For this review, use the dimensioned drawing (mm, ordinates from the lowest corner) and the shaded views. A direction names the side the tool comes from. Coordinates: 2 decimals unless noted, no trailing zeros. Loops run counter-clockwise (first coordinate to the right, second up) from the corner with the lowest first, then second, coordinate; pieces in that order, holes last. Notation, with made-up numbers: M 40.25,20.5 L 88.25,20.5 A30 cw 88.25,56.5 Z; hole C -39.5,41.5 d11. An arc over 180 degrees is marked long. Write item = value, one per line. Start each with the question number.
Q1. We need section D-D on z = 12.75. Give the boundary of the cut face in (x, y), and give its area (3 significant figures).
Q2. Mouldability with a two-part tool opening along Z and no side actions: class the marked faces 3 and 4 as released by +Z, released by -Z, zero draft, split by the parting line, or undercut.
Q3. We need section C-C on y = 4. Give the boundary of the cut face in (x, z), and give its area (3 significant figures).
Q4. We need section A-A on z = 8. Give the boundary of the cut face in (x, y).
Q5. We need section B-B on x = 30. Give the boundary of the cut face in (y, z).
Q6. Clearance check with flat-ended pins moving along their axes: pin 1 Ø2 at (x, z) = (11.5, 13) entering from -Y; pin 2 Ø6 at (y, z) = (27, 11.5) entering from +X; pin 3 Ø6 at (x, y) = (45, 13.5) entering from -Z. State where each tip first meets the part, or that it passes through.
Q7. Wall thickness on probe 1 along X at (y, z) = (15.5, 8); probe 2 along Y at (x, z) = (51.5, 8): over which ranges is each line inside the solid? List them lowest first.
Q8. For the marked faces 1 and 2, list the 3-axis set-ups (+Z, -Z, +X, -X, +Y, -Y) from which the entire face can be reached by the end or side of a thin tool; tool diameter is ignored.
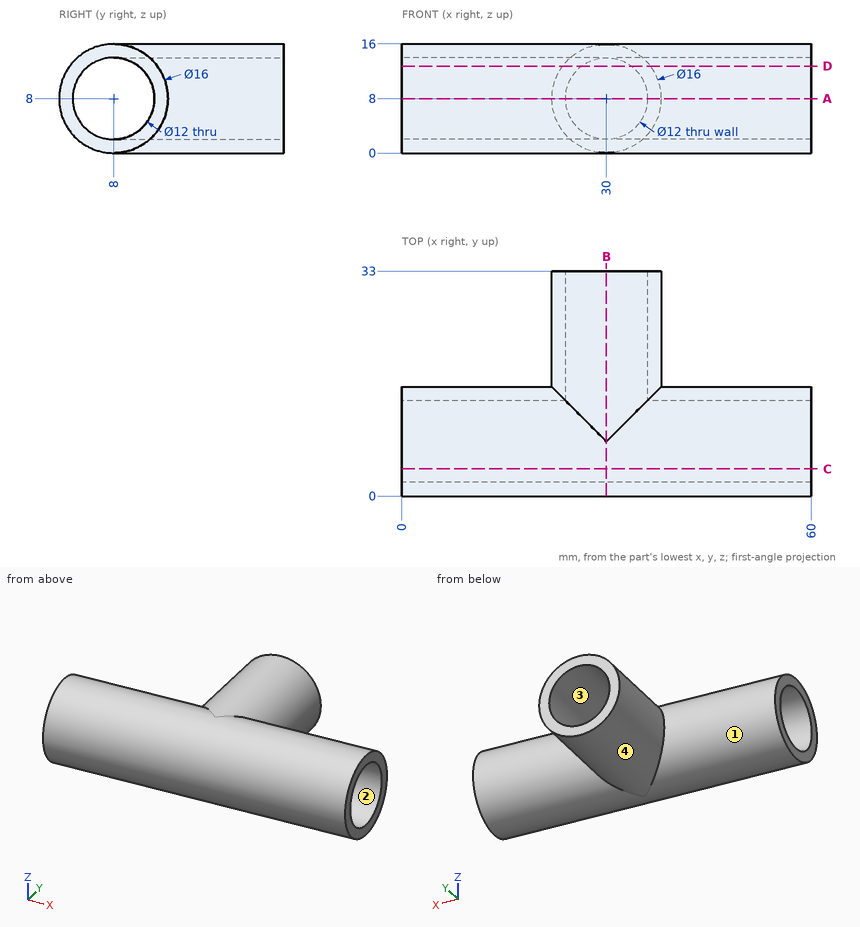
Returned:
q1.outline = M 0,1.56 L 60,1.56 L 60,4.33 L 0,4.33 Z; M 0,11.67 L 26.33,11.67 L 26.33,33 L 23.56,33 L 23.56,14.44 L 0,14.44 Z; M 33.67,11.67 L 60,11.67 L 60,14.44 L 36.44,14.44 L 36.44,33 L 33.67,33 Z
q1.area = 415 mm^2
q2.face_3 = undercut
q2.face_4 = split by the parting line
q3.outline = M 0,1.07 L 60,1.07 L 60,3.53 L 0,3.53 Z; M 0,12.47 L 60,12.47 L 60,14.93 L 0,14.93 Z
q3.area = 295 mm^2
q4.outline = M 0,0 L 60,0 L 60,2 L 0,2 Z; M 0,14 L 24,14 L 24,33 L 22,33 L 22,16 L 0,16 Z; M 36,14 L 60,14 L 60,16 L 38,16 L 38,33 L 36,33 Z
q5.outline = M 8,0 L 33,0 L 33,2 L 8,2 A6 cw 8,14 L 33,14 L 33,16 L 8,16 A8 ccw Z
q6.pin_1 = 1.07
q6.pin_2 = 37.98
q6.pin_3 = 0.4
q7.probe_1 = 0 to 24, 36 to 60
q7.probe_2 = 0 to 2, 14 to 16
q8.face_1 = none
q8.face_2 = +X, -X
